Read the model definition and answer for the solid it produces. Units are mm, in the model's axes. Face numbers are marked on the shaded views. A direction names the side the tool comes from. Coordinates: 2 decimals unless noted, no trailing zeros. Loops run counter-clockwise (first coordinate to the right, second up) from the corner with the lowest first, then second, coordinate; pieces in that order, holes last. Notation, with made-up numbers: (64.5, -6.75) - (118.5, -6.75) arc R21 cw to (118.5, 9.25) - close; hole circle Ø8 at (24, 87.5). An arc over 180 degrees is marked (long way). Use one line per item in the form item = value. Start each with the question number.
1) Which of the six approach directions +Z, -Z, +X, -X, +Y, -Y give full straight-line access (tool end or side, diameter ignored) to the marked faces 1, 2, 3, 4 and 5?
2) Consider line 1 (Y direction, x = 10, z = 5.5); line 2 (Y direction, x = 36.05, z = 3); line 3 (Z direction, x = 29, y = -28). Determine where each line is inside the solid, lowest interval first.
3) Each of these flat-tipped pins is pushed along its axis until it touches: P1, Ø3, axis at x = -11, z = 6, coming from the -Y side; P2, Ø2, axis at x = -11, z = 7, coming from the +Y side; P3, Ø12, axis at x = 75, y = 17.5, coming from the +Z side. Where does it stop, or does it pass through?
4) A cutting plane is placed at A-A (x = 50.25). Give the vertices of the cut face in (y, z), and give its area (3 significant figures).
5) A cutting plane is placed at D-D (y = 31.5). Give the vertices of the cut face in (x, z), and give its area (3 significant figures).
6) A cutting plane is placed at B-B (z = 3). State how many separate pieces and enclosed holes the cut face has, and give its area (3 significant figures).
7) A cutting plane is placed at C-C (y = -17.5). Give the vertices of the cut face in (x, z), and give its area (3 significant figures).
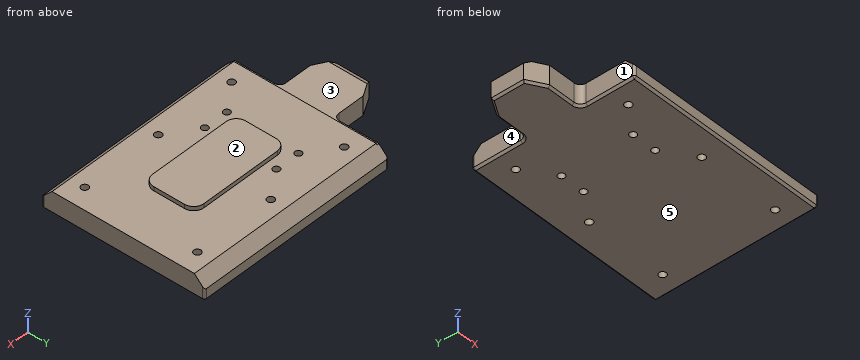
from build123d import *

# Parameters (mm, degrees)
BOSS_EXTRUDE1_DEPTH         = 12.7
CHAMFER1_SIZE               = 5
CHAMFER1_SIZE2              = 8.660254038
TAP_DRILL_FOR_M4X0_7_TAP1_D = 3.3
CUT_EXTRUDE2_START          = -2
CUT_EXTRUDE2_DEPTH          = 2
SKETCH6_W                   = 26
SKETCH6_H                   = 79.5
CUT_EXTRUDE1_DEPTH          = 0.5
FILLET1_R                   = 3
CHAMFER2_SIZE               = 1
CHAMFER3_SIZE               = 1.5
CHAMFER3_SIZE2              = 2.598076211
TAP_DRILL_FOR_M5X0_8_TAP1_D = 3.5
CHAMFER4_SIZE               = 5


# Some blends are built 0.0001 mm under size
with BuildPart() as part:
    # Sketch1 → Boss-Extrude1 (new body)
    with BuildSketch(Plane.XY):
        with BuildLine():
            Line((0, 38.75), (0, 12.9375))
            Line((0, 12.9375), (-25, 12.9375))
            Line((-25, 12.9375), (-25, -12.9375))
            Line((-25, -12.9375), (0, -12.9375))
            Line((0, -12.9375), (0, -38.75))
            ThreePointArc((0, -38.75), (0.292893219, -39.457106781), (1, -39.75))
            Line((1, -39.75), (99, -39.75))
            ThreePointArc((99, -39.75), (99.707106781, -39.457106781), (100, -38.75))
            Line((100, -38.75), (100, 38.75))
            ThreePointArc((100, 38.75), (99.707106781, 39.457106781), (99, 39.75))
            Line((99, 39.75), (1, 39.75))
            ThreePointArc((1, 39.75), (0.292893219, 39.457106781), (0, 38.75))
        make_face()
    extrude(amount=BOSS_EXTRUDE1_DEPTH)

    # Chamfer1
    chamfer1_edges = [part.edges().sort_by_distance(p)[0] for p in [
        (-25, -12.9375, 6.35),
        (-25, 12.9375, 6.35),
    ]]
    chamfer1_side = [part.faces().sort_by_distance(p)[0] for p in [
        (-25, 0, 6.35),
    ]]
    chamfer(chamfer1_edges, length=CHAMFER1_SIZE, length2=CHAMFER1_SIZE2, reference=chamfer1_side[0])

    # Tap Drill for M4x0.7 Tap1 (through all)
    with Locations(Plane(origin=(0, 0, 0), x_dir=(-1, 0, 0), z_dir=(0, 0, -1))):
        with Locations((-24.05, 17.5), (-24.05, -17.5), (-36.05, 17.5), (-36.05, -17.5)):
            Hole(TAP_DRILL_FOR_M4X0_7_TAP1_D / 2)

    # Sketch9 → Cut-Extrude2 (cut)
    with BuildSketch(Plane.XY.offset(12.7).offset(CUT_EXTRUDE2_START)):
        with BuildLine():
            Line((0, 12.9375), (-16.339745962, 12.9375))
            Line((-16.339745962, 12.9375), (-25, 7.9375))
            Line((-25, 7.9375), (-25, -7.9375))
            Line((-25, -7.9375), (-16.339745962, -12.9375))
            Line((-16.339745962, -12.9375), (0, -12.9375))
            Line((0, -12.9375), (0, -38.75))
            ThreePointArc((0, -38.75), (0.292893219, -39.457106781), (1, -39.75))
            Line((1, -39.75), (99, -39.75))
            ThreePointArc((99, -39.75), (99.707106781, -39.457106781), (100, -38.75))
            Line((100, -38.75), (100, 38.75))
            ThreePointArc((100, 38.75), (99.707106781, 39.457106781), (99, 39.75))
            Line((99, 39.75), (1, 39.75))
            ThreePointArc((1, 39.75), (0.292893219, 39.457106781), (0, 38.75))
            Line((0, 38.75), (0, 12.9375))
        make_face()
        with BuildLine():
            Line((70, -12.5), (30, -12.5))
            ThreePointArc((30, -12.5), (26.464466094, -11.035533906), (25, -7.5))
            Line((25, -7.5), (25, 7.5))
            ThreePointArc((25, 7.5), (26.464466094, 11.035533906), (30, 12.5))
            Line((30, 12.5), (70, 12.5))
            ThreePointArc((70, 12.5), (73.535533906, 11.035533906), (75, 7.5))
            Line((75, 7.5), (75, -7.5))
            ThreePointArc((75, -7.5), (73.535533906, -11.035533906), (70, -12.5))
        make_face(mode=Mode.SUBTRACT)
    extrude(amount=CUT_EXTRUDE2_DEPTH, mode=Mode.SUBTRACT)

    # Sketch6 → Cut-Extrude1 (cut)
    with BuildSketch(Plane.XY.offset(10.7)):
        with Locations((-12, 0)):
            Rectangle(SKETCH6_W, SKETCH6_H)
    extrude(amount=-CUT_EXTRUDE1_DEPTH, mode=Mode.SUBTRACT)

    # Fillet1
    fillet1_edges = [part.edges().sort_by_distance(p)[0] for p in [
        (0, 12.9375, 5.1),
        (0, -12.9375, 5.1),
    ]]
    fillet(fillet1_edges, radius=FILLET1_R)

    # Chamfer2
    chamfer2_edges = [part.edges().sort_by_distance(p)[0] for p in [
        (0, 27.34375, 0),
        (0.292893219, 39.457106781, 0),
        (50, 39.75, 0),
        (99.707106781, 39.457106781, 0),
        (100, 0, 0),
        (99.707106781, -39.457106781, 0),
        (50, -39.75, 0),
        (0.292893219, -39.457106781, 0),
        (0, -27.34375, 0),
        (-9.669872981, 12.9375, 0),
        (-0.878679656, -13.816179656, 0),
        (-0.878679656, 13.816179656, 0),
        (-25, 0, 0),
        (-9.669872981, -12.9375, 0),
        (-20.669872981, -10.4375, 0),
        (-20.669872981, 10.4375, 0),
    ]]
    chamfer(chamfer2_edges, length=CHAMFER2_SIZE - 0.0001)  # a hair under: the kernel refuses the full size

    # Chamfer3
    chamfer3_edges = [part.edges().sort_by_distance(p)[0] for p in [
        (-25, 0, 10.2),
    ]]
    chamfer3_side = [part.faces().sort_by_distance(p)[0] for p in [
        (-25, 0, 5.59995),
    ]]
    chamfer(chamfer3_edges, length=CHAMFER3_SIZE, length2=CHAMFER3_SIZE2, reference=chamfer3_side[0])

    # Tap Drill for M5x0.8 Tap1 (through all)
    with Locations(Plane(origin=(0, 0, 0), x_dir=(-1, 0, 0), z_dir=(0, 0, -1))):
        with Locations((-90.25, 27.5), (-50.25, 27.5), (-10.25, 27.5), (-10.25, -27.5), (-50.25, -27.5), (-90.25, -27.5)):
            Hole(TAP_DRILL_FOR_M5X0_8_TAP1_D / 2)

    # Chamfer4
    # the kernel refuses this chamfer: 5 mm, written as the material it takes off along each edge
    with BuildSketch(Plane(origin=(-11.85841494, -39.75, 10.7), x_dir=(0, -0.027495876610586317, -0.9996219169112968), z_dir=(1, 0, 0)), Plane(origin=(111.85841494, 39.75, 10.7), x_dir=(0, 0.027495876610586317, -0.9996219169112968), z_dir=(-1, 0, 0))) as chamfer4_piece_1:
        Polygon((CHAMFER4_SIZE * 0.999621916911, CHAMFER4_SIZE * 0.0274958766106), (-CHAMFER4_SIZE * 0.0274958766106, CHAMFER4_SIZE * 0.999621916911), (0, 0), align=None)
    extrude(amount=123.71682988, mode=Mode.SUBTRACT)


solid = part.part
Found:
q1.face_1 = +Z, -Z, -X, -Y
q1.face_2 = +Z, +X, -X, +Y, -Y
q1.face_3 = +Z, -X, +Y, -Y
q1.face_4 = +Z, -Z, -X, +Y
q1.face_5 = -Z, +X, -X, +Y, -Y
q2.line_1 = -39.75 to -29.23, -25.77 to 25.77, 29.23 to 39.75
q2.line_2 = -39.75 to -19.15, -15.85 to 15.85, 19.15 to 39.75
q2.line_3 = 0 to 10.7
q3.P1 = -12.94
q3.P2 = 12.94
q3.P3 = 10.7
q4.outline = (-39.75, 1) - (-38.75, 0) - (-29.25, 0) - (-29.25, 10.7) - (-34.75, 10.7) - (-39.75, 5.7) - close; (-25.75, 0) - (25.75, 0) - (25.75, 10.7) - (12.5, 10.7) - (12.5, 12.7) - (-12.5, 12.7) - (-12.5, 10.7) - (-25.75, 10.7) - close; (29.25, 0) - (38.75, 0) - (39.75, 1) - (39.75, 5.7) - (34.75, 10.7) - (29.25, 10.7) - close
q4.area = 800 mm^2
q5.outline = (0, 1) - (1, 0) - (99, 0) - (100, 1) - (100, 10.7) - (1, 10.7) - (1, 10.2) - (0, 10.2) - close
q5.area = 1,070 mm^2
q6.separate_pieces = 1
q6.enclosed_holes = 10
q6.area = 8,460 mm^2
q7.outline = (0, 1) - (1, 0) - (22.4, 0) - (22.4, 10.7) - (1, 10.7) - (1, 10.2) - (0, 10.2) - close; (25.7, 0) - (34.4, 0) - (34.4, 10.7) - (25.7, 10.7) - close; (37.7, 0) - (99, 0) - (100, 1) - (100, 10.7) - (37.7, 10.7) - close
q7.area = 998 mm^2
